Build history of the part. All positions in model axes, mm. Face numbers are marked on the shaded views. A direction names the side the tool comes from. Round coordinates to 2 decimals unless told otherwise and drop trailing zeros. Write each loop counter-clockwise with the first axis right and the second up, starting at its lowest first coordinate (ties: lowest second). Pieces come first, ordered by that corner, then holes.
Item 1: Drop flat-ended pins along their axis: pin 1 Ø1 at (x, y) = (-4.5, 9.5) entering from +Z; pin 2 Ø5.5 at (x, y) = (0, 0) entering from -Z; pin 3 Ø1 at (x, z) = (0.5, 3.5) entering from +Y (3 decimals); pin 4 Ø1 at (y, z) = (6.5, 3) entering from +X. Give the stop position or say it passes through.
Item 2: Band-saw the part on B-B, the plane y = 5. Write the cut outline in (x, z) (3 decimals), then the cut area to 3 significant figures.
Item 3: Wall check: probe 1 along X at (y, z) = (0, 0.35) (3 decimals); probe 2 along Z at (x, y) = (3.25, -0.5); probe 3 along X at (y, z) = (2.5, 1). Give the ranges that are in metal, low to high.
Item 4: Mould opens along X. For the marked faces 1, 2 and 3 say: +X half, -X half, draft (parallel to the pull), parting line (faces both ways), or undercut.
Item 5: Band-saw the part on A-A, the plane x = 0. Write the cut outline in (y, z) (1 decimal).
Item 6: 3-axis set-ups, long thin cutter, end or side, ignore diameter. For the marked faces 4, 5, 6, 7 and 8: which of +Z, -Z, +X, -X, +Y, -Y reach the whole face in a straight line?
Item 7: Band-saw the part on D-D, the plane y = 8. Write the cut outline in (x, z) (1 decimal), then the cut area to 3 significant figures.
Autodesk Inventor part; units mm, degrees
ref_plane "Work Plane1" through (0, 0, 6.35) normal (0, 0, 1) x (1, 0, 0)
ref_plane "YZ Plane" through (0, 0, 0) normal (1, 0, 0) x (0, 1, 0)
ref_plane "XZ Plane" through (0, 0, 0) normal (0, 1, 0) x (-1, 0, 0)
sketch "Sketch1" plane through (0, 0, 0) normal (0, 0, 1) x (1, 0, 0)
  circle A0 centre (0, 0) radius 4.445
  line L0 (0, 0) -> (0, 12.7)
  line L1 (0, 12.7) -> (-2.54, 12.7)
  line L2 (-2.54, 12.7) -> (2.54, 12.7)
  line L3 (-2.54, 12.7) -> (-4.3931, 0.6771)
  line L4 (2.54, 12.7) -> (4.3931, 0.6771)
  line L5 (-2.54, 12.7) -> (-5.08, 12.7)
  line L6 (-5.08, 12.7) -> (-6.985, 0)
  line L7 (-6.985, 0) -> (-4.445, 0)
  line L8 (2.54, 12.7) -> (5.08, 12.7)
  line L9 (5.08, 12.7) -> (6.985, 0)
  line L10 (6.985, 0) -> (4.445, 0)
  arc A1 (-6.985, 0) -> (6.985, 0) centre (0, 0) ccw
  dimension "d0" = 8.89
  dimension "d1" = 12.7
  dimension "d2" = 2.54
  dimension "d3" = 5.08
  dimension "d4" = 2.54
  dimension "d5" = 2.54
  dimension "d6" = 2.54
  dimension "d7" = 2.54
extrude "Extrusion1" add sketch "Sketch1" along normal blind 1.5875 contours L10 A1 L7 A0 | A0 L4 L8 L9 L10 | L7 L6 L5 L3 A0
sketch "Sketch2" plane through (0, 0, 1.5875) normal (0, 0, 1) x (1, 0, 0)
  line L0 (-2.54, 12.7) -> (-5.08, 12.7)
  line L1 (-5.08, 12.7) -> (-6.985, 0)
  arc A0 (-6.985, 0) -> (6.985, 0) centre (0, 0) ccw
  line L2 (6.985, 0) -> (5.08, 12.7)
  line L3 (5.08, 12.7) -> (2.54, 12.7)
  line L4 (2.54, 12.7) -> (4.3931, 0.6771)
  arc A1 (-4.3931, 0.6771) -> (4.3931, 0.6771) centre (0, 0) ccw
  line L5 (-4.3931, 0.6771) -> (-2.54, 12.7)
  line L6 (-6.5088, 3.175) -> (6.5087, 3.175)
  dimension "d18" = 3.175
ref_plane "Work Plane1" through (0, 0, 6.35) normal (0, 0, 1) x (1, 0, 0)
extrude "Extrusion4" add sketch "Sketch2" along normal blind 3.175 contours L6 L4 A1 L5 | L5 A1 L4 L6 L2 A0 L1
sketch "Sketch4" plane through (0, 0, 4.7625) normal (0, 0, 1) x (1, 0, 0)
  line L0 (-1.8034, 1.0795) -> (1.8034, 1.0795)
  line L1 (1.8034, 1.0795) -> (1.8034, -1.0795)
  line L2 (1.8034, -1.0795) -> (-1.8034, -1.0795)
  line L3 (-1.8034, -1.0795) -> (-1.8034, 1.0795)
  arc A0 (-6.985, 0) -> (6.985, 0) centre (0, 0) ccw
  point P0 (0, 0)
  dimension "d23" = 3.6068
  dimension "d24" = 2.159
  dimension "d25" = 1.8034
  dimension "d26" = 1.0795
extrude "Extrusion6" cut sketch "Sketch4" against normal blind 3.175
fillet "Fillet1" radius 3.175 2 edges at (-5.2584, 3.175, 1.5875) (5.2584, 3.175, 1.5875)
fillet "Fillet2" radius 0.762 3 edges at (-4.2006, 1.9261, 1.5875) (4.2006, 1.9261, 1.5875) (0, -4.445, 1.5875)
properties part number "servoPotentiometerAttachment" material "ABS Plastic"
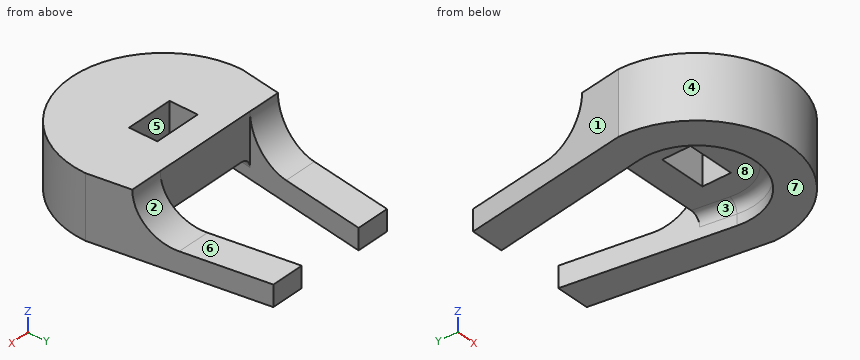
Results:
1. pin 1: stops at z = 1.59
1. pin 2: stops at z = 1.59
1. pin 3: stops at y = 3.175
1. pin 4: passes through
2. outline: (-6.235, 0) - (-3.727, 0) - (-3.727, 1.889) - (-6.235, 1.889) - close; (3.727, 0) - (6.235, 0) - (6.235, 1.889) - (3.727, 1.889) - close
2. area: 9.47 mm2
3. probe 1: x = -6.985 to -4.445, 4.445 to 6.985
3. probe 2: z = 1.59 to 4.76
3. probe 3: x = -6.61 to -4.09, 4.09 to 6.61
4. face 1: -X half
4. face 2: draft
4. face 3: undercut
5. outline: (-7, 0) - (-4.4, 0) - (-4.4, 0.8) arc R0.8 cw to (-3.7, 1.6) - (-1.1, 1.6) - (-1.1, 4.8) - (-7, 4.8) - close; (1.1, 1.6) - (3.2, 1.6) - (3.2, 4.8) - (1.1, 4.8) - close
6. face 4: +Z, -Z, -Y
6. face 5: +Z, -Z
6. face 6: +Z, +X, -X, +Y
6. face 7: -Z, +X, -X, +Y, -Y
6. face 8: -Z
7. outline: (-5.8, 0) - (-3.3, 0) - (-3.3, 1.6) - (-5.8, 1.6) - close; (3.3, 0) - (5.8, 0) - (5.8, 1.6) - (3.3, 1.6) - close
7. area: 8.00 mm2
